Check sheet for the modelled part. Datum: model origin and axes. Units: mm. Face numbers are marked on the shaded views. A direction names the side the tool comes from. Give positions to 0.01 mm unless a question says otherwise; leave off trailing zeros. Loops run counter-clockwise (first coordinate to the right, second up) from the corner with the lowest first, then second, coordinate; pieces in that order, holes last. Notation, with made-up numbers: (23, 81.25) - (58, 81.25) arc R31 ccw to (58, 116.25) - close; hole circle Ø11 at (80.25, -34). An arc over 180 degrees is marked (long way). Answer in a Markdown table with one row per item. Add a question column.
(1) Go/stop test with flat-tipped pins: P1, Ø3, axis at y = 0, z = 0, coming from the -X side; P2, Ø10, axis at y = -12, z = 15.5, coming from the -X side; P3, Ø5, axis at x = -5.5, z = -1.5, coming from the +Y side; P4, Ø10, axis at x = -40, z = -9.5, coming from the -Y side. Record where each tip stops, or that it passes through.
(2) Thickness scan on L1, parallel to Y at x = 5, z = 0; L2, parallel to X at y = -1, z = -16; L3, parallel to Y at x = -40.5, z = 0. Record the ranges inside material, lowest first.
(3) Set-up check for the marked faces 1 and 2: record each of +Z, -Z, +X, -X, +Y, -Y from which the full face is reachable in a straight line by a thin tool's end or side.
(4) Sectioned sample at B-B on x = -35.5. Enter the section's corners in (y, z).
(5) Sectioned sample at A-A on x = -79. Enter the section's corners in (y, z), then the cut area to 3 significant figures.
from build123d import *


with BuildPart() as part:
    # Axial profile (mm) → Full revolution (revolve)
    with BuildSketch(Plane.XY, mode=Mode.PRIVATE) as full_revolution_sk:
        Polygon((-94, 2.4), (58, 2.4), (58, 3.2), (13, 3.2), (13, 6), (0, 6), (0, 20), (-2, 20), (-5, 17), (-5, 7.9), (-19, 7.9), (-19, 5.7), (-23, 5.7), (-23, 6.7), (-27, 6.7), (-27, 6.4), (-49, 6.4), (-49, 3.2), (-94, 3.2), align=None)
    revolve(full_revolution_sk.sketch.rotate(Axis((-110, 0, 0), (1, 0, 0)), 90), axis=Axis((-110, 0, 0), (1, 0, 0)))


solid = part.part
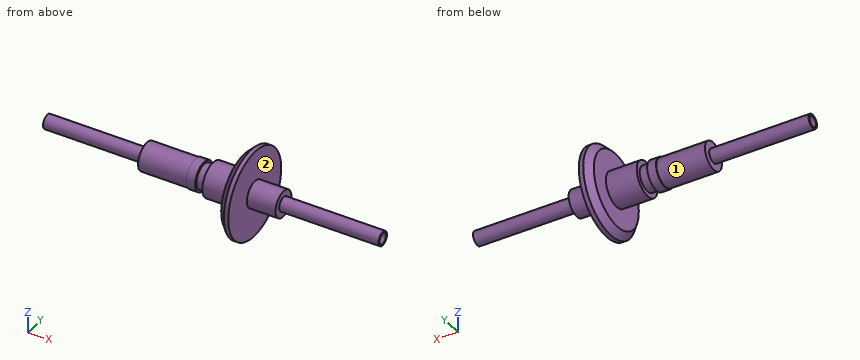
Reply:
| question | item | result |
|---|---|---|
| 1 | P1 | through |
| 1 | P2 | x = -5 |
| 1 | P3 | y = 18.95 |
| 1 | P4 | y = -4.55 |
| 2 | L1 | -6 to -2.4, 2.4 to 6 |
| 2 | L2 | -5 to 0 |
| 2 | L3 | -6.4 to -2.4, 2.4 to 6.4 |
| 3 | face 1 | -X |
| 3 | face 2 | +X |
| 4 | outline | circle Ø12.8 at (0, 0); hole circle Ø4.8 at (0, 0) |
| 5 | outline | circle Ø6.4 at (0, 0); hole circle Ø4.8 at (0, 0) |
| 5 | area | 14.1 mm^2 |
